```python
from build123d import *

# Parameters (mm, degrees)
SKETCH1_W           = 139
SKETCH1_H           = 90
SKETCH1_R           = 1.6
SKETCH1_R_2         = 3.75
SKETCH1_R_3         = 3.1
SKETCH1_W_2         = 2.2
SKETCH1_H_2         = 1.1
SKETCH1_W_3         = 1.2
SKETCH1_H_3         = 2.7
SKETCH1_W_4         = 3.2
SKETCH1_H_4         = 1.9
BOSS_EXTRUDE1_DEPTH = 3


with BuildPart() as part:
    # Sketch1 → Boss-Extrude1 (new body)
    with BuildSketch(Plane.XY):
        with Locations((69.5, 45)):
            Rectangle(SKETCH1_W, SKETCH1_H)
        with Locations((4, 79.5)):
            Circle(SKETCH1_R, mode=Mode.SUBTRACT)
        with Locations((135, 79.5)):
            Circle(SKETCH1_R, mode=Mode.SUBTRACT)
        with Locations((135, 13.5)):
            Circle(SKETCH1_R, mode=Mode.SUBTRACT)
        with Locations((4, 13.5)):
            Circle(SKETCH1_R, mode=Mode.SUBTRACT)
        with Locations((15, 64.814177958)):
            Circle(SKETCH1_R, mode=Mode.SUBTRACT)
        with Locations((38.235051241, 71.614177958)):
            Circle(SKETCH1_R_2, mode=Mode.SUBTRACT)
        with Locations((124, 27.251424775)):
            Circle(SKETCH1_R, mode=Mode.SUBTRACT)
        with Locations((24.931997534, 16.841976033)):
            Circle(SKETCH1_R_2, mode=Mode.SUBTRACT)
        with Locations((52.931997534, 16.841976033)):
            Circle(SKETCH1_R_2, mode=Mode.SUBTRACT)
        with Locations((80.931997534, 16.841976033)):
            Circle(SKETCH1_R_2, mode=Mode.SUBTRACT)
        with Locations((114.931997534, 16.841976033)):
            Circle(SKETCH1_R_2, mode=Mode.SUBTRACT)
        with Locations((69.5, 71.675460618)):
            Circle(SKETCH1_R_3, mode=Mode.SUBTRACT)
        with Locations((113.751643049, 71.275460618)):
            Circle(SKETCH1_R_2, mode=Mode.SUBTRACT)
        with Locations((69.5, 45)):
            Circle(SKETCH1_R, mode=Mode.SUBTRACT)
        with Locations((38.235051241, 65.364177958)):
            Rectangle(SKETCH1_W_2, SKETCH1_H_2, mode=Mode.SUBTRACT)
        with Locations((24.931997534, 10.591976033)):
            Rectangle(SKETCH1_W_2, SKETCH1_H_2, mode=Mode.SUBTRACT)
        with Locations((52.931997534, 10.591976033)):
            Rectangle(SKETCH1_W_2, SKETCH1_H_2, mode=Mode.SUBTRACT)
        with Locations((80.931997534, 10.591976033)):
            Rectangle(SKETCH1_W_2, SKETCH1_H_2, mode=Mode.SUBTRACT)
        with Locations((114.931997534, 10.591976033)):
            Rectangle(SKETCH1_W_2, SKETCH1_H_2, mode=Mode.SUBTRACT)
        with BuildLine():
            Line((97.198408737, 42.05), (101.325150794, 42.05))
            ThreePointArc((101.325150794, 42.05), (102.861779766, 45), (101.325150794, 47.95))
            Line((101.325150794, 47.95), (97.198408737, 47.95))
            ThreePointArc((97.198408737, 47.95), (95.661779766, 45), (97.198408737, 42.05))
        make_face(mode=Mode.SUBTRACT)
        with Locations((75.5, 71.675460618)):
            Rectangle(SKETCH1_W_3, SKETCH1_H_3, mode=Mode.SUBTRACT)
        with Locations((113.751643049, 78.975460618)):
            Rectangle(SKETCH1_W_4, SKETCH1_H_4, mode=Mode.SUBTRACT)
        with BuildLine():
            Line((21.768626506, 42.05), (25.895368563, 42.05))
            ThreePointArc((25.895368563, 42.05), (27.431997534, 45), (25.895368563, 47.95))
            Line((25.895368563, 47.95), (21.768626506, 47.95))
            ThreePointArc((21.768626506, 47.95), (20.231997534, 45), (21.768626506, 42.05))
        make_face(mode=Mode.SUBTRACT)
    extrude(amount=BOSS_EXTRUDE1_DEPTH)


solid = part.part
```
The listing builds one solid part. Answer for the finished solid, in the listing's coordinates (mm). A direction names the side the tool comes from. Coordinates: 2 decimals unless noted, no trailing zeros. Order: outer loops, then holes, each group sorted by start corner. A loop starts at its lowest first (then second) coordinate and runs counter-clockwise, first axis right, second up. Notation, with made-up numbers: M 16.25,72 L 49.25,72 A19 ccw 49.25,93 Z; hole C 88.25,23.5 d4. An arc over 180 degrees is marked long. Answer as a JSON object with one key per item and string values. Group by question number.
1. Section C-C on y = 45 is taken. Write down the section's boundary in (x, z).
2. Section B-B on x = 124 is taken. Write down the section's boundary in (y, z).
3. Section D-D on x = 4 is taken. Write down the section's boundary in (y, z).
4. A tool of negligible diameter and unlimited length cuts with its end or side. For faces 1 (the flat face through (99, 42.05, 1)), 2 (the flat face through (69, 0, 1)), from which of +Z, -Z, +X, -X, +Y, -Y can it reach the whole face along a straight path? Write none if from no direction.
5. Determine the mould class of faces 3 (the flat face through (114, 79.925, 1)), 4 (the flat face through (139, 44, 1)), 5 (the flat face through (69, 56, 3)), 6 (the cylindrical face through (3.792, 81.086, 1.479)) for opening direction X: released by +X, released by -X, zero draft, split by the parting line, or undercut.
6. Section A-A on x = 69.5 is taken. Write down the section's boundary in (y, z), then the cut area to 3 significant figures.
7. Straight lines are drawn through the part: line 1 (Y direction, x = 69.5, z = 1); line 2 (Y direction, x = 100.5, z = 1.4); line 3 (X direction, y = 46, z = 1.65). For each, find the intervals that lie inside material, in ascending order.
Values follow:
{
 "1": {"outline": "M 0,0 L 20.23,0 L 20.23,3 L 0,3 Z; M 27.43,0 L 67.9,0 L 67.9,3 L 27.43,3 Z; M 71.1,0 L 95.66,0 L 95.66,3 L 71.1,3 Z; M 102.86,0 L 139,0 L 139,3 L 102.86,3 Z"},
 "2": {"outline": "M 0,0 L 25.65,0 L 25.65,3 L 0,3 Z; M 28.85,0 L 90,0 L 90,3 L 28.85,3 Z"},
 "3": {"outline": "M 0,0 L 11.9,0 L 11.9,3 L 0,3 Z; M 15.1,0 L 77.9,0 L 77.9,3 L 15.1,3 Z; M 81.1,0 L 90,0 L 90,3 L 81.1,3 Z"},
 "4": {"face 1": "+Z, -Z", "face 2": "+Z, -Z, +X, -X, -Y"},
 "5": {"face 3": "undercut", "face 4": "released by +X", "face 5": "zero draft", "face 6": "undercut"},
 "6": {"outline": "M 0,0 L 43.4,0 L 43.4,3 L 0,3 Z; M 46.6,0 L 68.58,0 L 68.58,3 L 46.6,3 Z; M 74.78,0 L 90,0 L 90,3 L 74.78,3 Z", "area": "242 mm2"},
 "7": {"line 1": "0 to 43.4, 46.6 to 68.58, 74.78 to 90", "line 2": "0 to 42.05, 47.95 to 90", "line 3": "0 to 20.37, 27.29 to 68.25, 70.75 to 95.8, 102.72 to 139"}
}
